Geometry check sheet. Reference: drawing and pictorial views, mm from the part's lowest x, y, z. Coordinates: 2 decimals unless noted, no trailing zeros. Write each loop counter-clockwise with the first axis right and the second up, starting at its lowest first coordinate (ties: lowest second). Pieces come first, ordered by that corner, then holes. Notation, with made-up numbers: (74, -29) -> (90, -29) arc R22 ccw to (90, -15) -> close; hole circle Ø8 at (-4.75, -21). An arc over 180 degrees is marked (long way). Use a Markdown table: item, result. Add a question column.
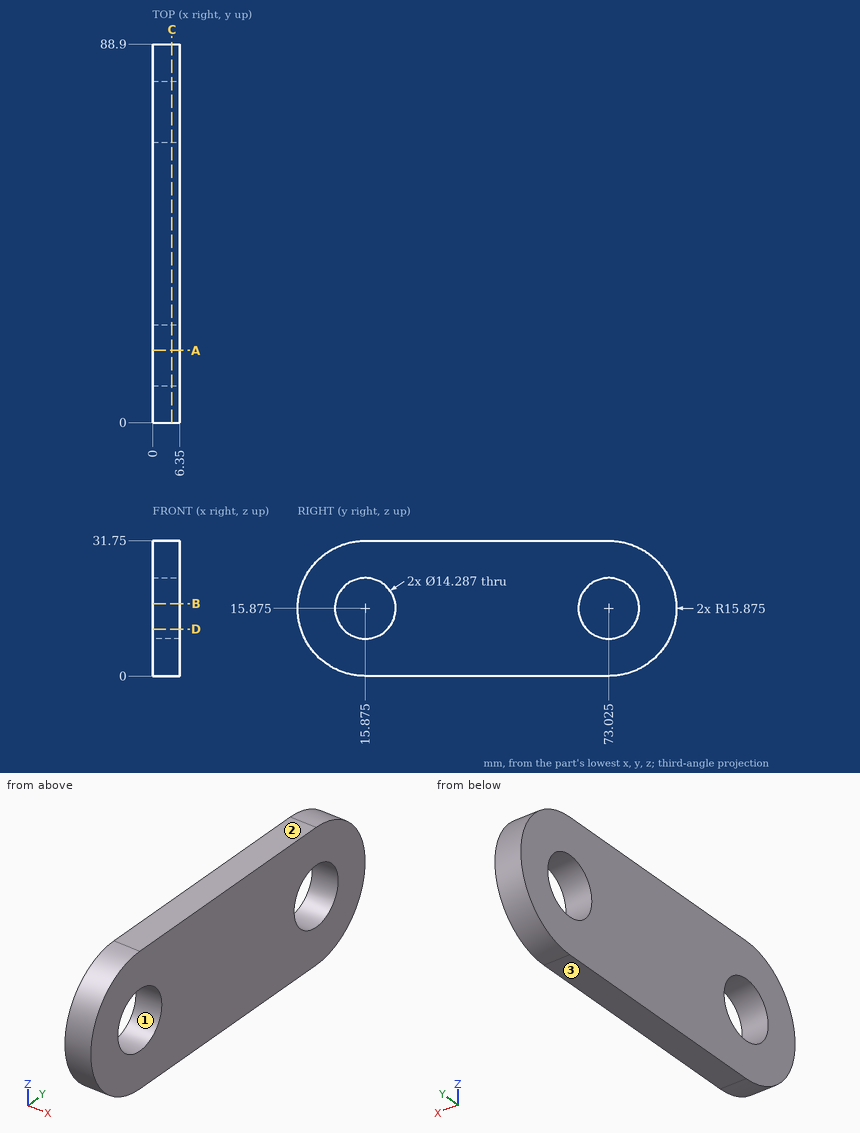
1) Cross-section at B-B on z = 17. Record the boundary of the cut face in (x, y), then the cut area to 3 significant figures.
2) Cross-section at D-D on z = 11. Record the boundary of the cut face in (x, y), then the cut area to 3 significant figures.
3) Cross-section at A-A on y = 17. Record the boundary of the cut face in (x, z), then the cut area to 3 significant figures.
4) Release check for a two-part mould opening along Z. For the marked faces 1, 2 and 3 record: released by +Z, released by -Z, zero draft, split by the parting line, or undercut.
5) Gauge pin test, flat ends, axial feed: pin 1 (1.5 mm diameter, centred on x = 1, z = 27.5, fed in from -Y); pin 2 (2 mm diameter, centred on x = 4.5, z = 9.5, fed in from -Y); pin 3 (1.5 mm diameter, centred on x = 5.5, y = 9.5, fed in from -Z). Record the tip position at first contact, or that the pin passes through.
6) Cross-section at C-C on x = 4.5. Give the number of separate pieces and of enclosed holes in the cut face, then the cut area to 3 significant figures.
7) Thickness scan on L1, parallel to Y at x = 5.25, z = 16; L2, parallel to Y at x = 5.75, z = 20 (1 decimal); L3, parallel to Z at x = 6, y = 76. Record the ranges inside material, lowest first.
Returned:
| question | item | result |
|---|---|---|
| 1 | outline | (0, 0.04) -> (6.35, 0.04) -> (6.35, 8.82) -> (0, 8.82) -> close; (0, 22.93) -> (6.35, 22.93) -> (6.35, 65.97) -> (0, 65.97) -> close; (0, 80.08) -> (6.35, 80.08) -> (6.35, 88.86) -> (0, 88.86) -> close |
| 1 | area | 385 mm² |
| 2 | outline | (0, 0.77) -> (6.35, 0.77) -> (6.35, 10.65) -> (0, 10.65) -> close; (0, 21.1) -> (6.35, 21.1) -> (6.35, 67.8) -> (0, 67.8) -> close; (0, 78.25) -> (6.35, 78.25) -> (6.35, 88.13) -> (0, 88.13) -> close |
| 2 | area | 422 mm² |
| 3 | outline | (0, 0) -> (6.35, 0) -> (6.35, 8.82) -> (0, 8.82) -> close; (0, 22.93) -> (6.35, 22.93) -> (6.35, 31.75) -> (0, 31.75) -> close |
| 3 | area | 112 mm² |
| 4 | face 1 | undercut |
| 4 | face 2 | released by +Z |
| 4 | face 3 | released by -Z |
| 5 | pin 1 | stops at y = 4.31 |
| 5 | pin 2 | stops at y = 0.94 |
| 5 | pin 3 | stops at z = 1.03 |
| 6 | separate pieces | 1 |
| 6 | enclosed holes | 2 |
| 6 | area | 2,290 mm² |
| 7 | L1 | y = 0 to 8.73, 23.02 to 65.88, 80.17 to 88.9 |
| 7 | L2 | y = 0.5 to 10, 21.7 to 67.2, 78.9 to 88.4 |
| 7 | L3 | z = 0.28 to 9.38, 22.37 to 31.47 |
